Here's how the part is built. I have some questions about the finished solid (model axes, mm). A direction names the side the tool comes from. Coordinates: 2 decimals unless noted, no trailing zeros. Write each loop counter-clockwise with the first axis right and the second up, starting at its lowest first coordinate (ties: lowest second). Pieces come first, ordered by that corner, then holes. Notation, with made-up numbers: M 76.5,-33 L 96.5,-33 A12 cw 96.5,-29 Z; hole C 75,-26 d7. An arc over 180 degrees is marked long. Use one line per item in the form item = value. Start each with the question number.
1. I want a section at C-C, the plane z = 0. List the corners of the cut face in (x, y) for me, plus the area to 3 significant figures.
2. I'm going to push flat-ended pins straight in: pin 1 Ø6 at (y, z) = (-15, 7.5) entering from -X; pin 2 Ø8 at (y, z) = (5.5, 7.5) entering from -X; pin 3 Ø2 at (x, z) = (-162.5, -12) entering from +Y. Where does each tip first touch, or does it pass through?
3. On a 3-axis mill with a long thin cutter (end or side, diameter ignored), from which of +Z, -Z, +X, -X, +Y, -Y can I reach the whole of each face in a straight line? I mean faces 5 (the face through (205, 0, 0)), 6 (the face through (-198, 0.3, -10.2)), 7 (the face through (199.01, -9.76, 2.17)). Say none if no direction works.
4. Please list where these lines run through material, in increasing order: line 1 along Y through (x, z) = (0, -5.75); line 2 along X through (y, z) = (-7.5, 5.25); line 3 along X through (y, z) = (-15.5, -3.5). Write a range as [from, to].
5. I want a section at A-A, the plane y = 0. List the corners of the cut face in (x, z) for me, plus the area to 3 significant figures.
6. Thinking about a two-plate mould opening in Y: for faces 1 (the face through (-3, -20, 0)), 2 (the face through (-200, -2, -5)), 3 (the face through (-1.172, 8.923, 0.21)), 4 (the face through (-198.99, -9.76, 2.17)), which applies, released by +Y, released by -Y, zero draft, split by the parting line, or undercut?
7. I want a section at B-B, the plane x = 0. List the corners of the cut face in (y, z) for me, plus the area to 3 significant figures.
from build123d import *

# Parameters (mm, degrees)
SKETCH1_R           = 10
BOSS_EXTRUDE1_DEPTH = 205
SKETCH2_R           = 12.5
SKETCH2_R_2         = 5
CUT_EXTRUDE1_DEPTH  = 5
SKETCH3_W           = 40
SKETCH3_H           = 40
BOSS_EXTRUDE5_DEPTH = 15
SKETCH4_R           = 9
CUT_EXTRUDE2_DEPTH  = 15
FILLET2_R           = 2
SKETCH5_W           = 30
SKETCH5_H           = 40
BOSS_EXTRUDE6_DEPTH = 178
SKETCH6_W           = 30
SKETCH6_H           = 40
BOSS_EXTRUDE7_DEPTH = 178
FILLET3_R           = 5


with BuildPart() as part:
    # Sketch1 → Boss-Extrude1 (new body, symmetric)
    with BuildSketch(Plane(origin=(0, 0, 0), x_dir=(0, 0, -1), z_dir=(1, 0, 0))):
        Circle(SKETCH1_R)
    extrude(amount=BOSS_EXTRUDE1_DEPTH, both=True)

    # Sketch2 → Cut-Extrude1 (cut)
    with BuildSketch(Plane.ZY.offset(205)):
        Circle(SKETCH2_R)
        Circle(SKETCH2_R_2, mode=Mode.SUBTRACT)
    cut_extrude1 = extrude(amount=-CUT_EXTRUDE1_DEPTH, mode=Mode.SUBTRACT)

    # Mirror1: Cut-Extrude1 across plane
    add(cut_extrude1.mirror(Plane(origin=(0, 0, 0), x_dir=(0, 0, 1), z_dir=(1, 0, 0))), mode=Mode.SUBTRACT)

    # Sketch3 → Boss-Extrude5 (add, symmetric)
    with BuildSketch(Plane.XY):
        Rectangle(SKETCH3_W, SKETCH3_H)
    extrude(amount=BOSS_EXTRUDE5_DEPTH, both=True)

    # Sketch4 → Cut-Extrude2 (cut, symmetric)
    with BuildSketch(Plane.XY):
        Circle(SKETCH4_R)
    extrude(amount=CUT_EXTRUDE2_DEPTH, both=True, mode=Mode.SUBTRACT)

    # Fillet2
    fillet2_edges = [part.edges().sort_by_distance(p)[0] for p in [
        (-20, 0, 10),
        (20, 0, 10),
    ]]
    fillet(fillet2_edges, radius=FILLET2_R)

    # Sketch5 → Boss-Extrude6 (add)
    with BuildSketch(Plane.ZY.offset(20)):
        Rectangle(SKETCH5_W, SKETCH5_H)
    extrude(amount=BOSS_EXTRUDE6_DEPTH)

    # Sketch6 → Boss-Extrude7 (add)
    with BuildSketch(Plane(origin=(20, 0, 0), x_dir=(0, 0, -1), z_dir=(1, 0, 0))):
        Rectangle(SKETCH6_W, SKETCH6_H)
    extrude(amount=BOSS_EXTRUDE7_DEPTH)

    # Fillet3
    fillet3_edges = [part.edges().sort_by_distance(p)[0] for p in [
        (0, -20, -15),
        (0, 20, 15),
        (0, -20, 15),
        (0, 20, -15),
    ]]
    fillet(fillet3_edges, radius=FILLET3_R)


solid = part.part
Answer list:
q1.outline = M -205,-5 L -200,-5 L -200,-10 L -198,-10 L -198,-20 L 198,-20 L 198,-10 L 200,-10 L 200,-5 L 205,-5 L 205,5 L 200,5 L 200,10 L 198,10 L 198,20 L -198,20 L -198,10 L -200,10 L -200,5 L -205,5 Z; hole C 0,0 d18
q1.area = 15,800 mm²
q2.pin_1 = -198
q2.pin_2 = -200
q2.pin_3 = 19.9
q3.face_5 = +Z, -Z, +X, +Y, -Y
q3.face_6 = -X
q3.face_7 = +X
q4.line_1 = [-20, -9], [9, 20]
q4.line_2 = [-200, -4.97], [4.97, 200]
q4.line_3 = [-198, 198]
q5.outline = M -205,-5 L -200,-5 L -200,-10 L -198,-10 L -198,-15 L -9,-15 L -9,15 L -198,15 L -198,10 L -200,10 L -200,5 L -205,5 Z; M 9,-15 L 198,-15 L 198,-10 L 200,-10 L 200,-5 L 205,-5 L 205,5 L 200,5 L 200,10 L 198,10 L 198,15 L 9,15 Z
q5.area = 11,500 mm²
q6.face_1 = released by -Y
q6.face_2 = zero draft
q6.face_3 = undercut
q6.face_4 = split by the parting line
q7.outline = M -20,-10 A5 ccw -15,-15 L -9,-15 L -9,15 L -15,15 A5 ccw -20,10 Z; M 9,-15 L 15,-15 A5 ccw 20,-10 L 20,10 A5 ccw 15,15 L 9,15 Z
q7.area = 639 mm²
